Design review of the part built by this model. Coordinates are the model's own, in mm. A direction names the side the tool comes from. Round coordinates to 2 decimals unless told otherwise and drop trailing zeros. Loops run counter-clockwise (first coordinate to the right, second up) from the corner with the lowest first, then second, coordinate; pieces in that order, holes last. Notation, with made-up numbers: (56, 30) - (83, 30) arc R34 ccw to (83, 69) - close; hole circle Ø3 at (0, 39). An arc over 180 degrees is marked (long way). Use one line per item in the form item = value. Start each with the question number.
(1) We need section B-B, the plane z = 0. Write out the cut boundary in (x, y), then the cut area to 3 significant figures.
(2) We need section D-D, the plane y = 0.5. Write out the cut boundary in (x, z) (1 decimal), then the cut area to 3 significant figures.
(3) Wall thickness on probe 1 along Z at (x, y) = (6, -2.75) (3 decimals); probe 2 along Z at (x, y) = (1, -3) (3 decimals); probe 3 along X at (y, z) = (-4.25, 1): over which ranges is each line inside the solid? List them lowest first. Write a range as [from, to].
(4) For pin 1 (2 mm diameter, centred on y = -2.5, z = 6, fed in from +X); pin 2 (2 mm diameter, centred on x = 0, z = 0.5, fed in from -Y), all flat-tipped, find the tip position at first contact; note any pin that passes through.
(5) Machinability: for faces 1 (the cylindrical face through (12.362, -2.929, -7.521)), 2 (the flat face through (-12.588, -3, 0)), which of the approach directions +Z, -Z, +X, -X, +Y, -Y give a long, thin tool a straight path to every point of the face, cutting with its end or side? Answer none if there is none.
(6) The part is to be moulded in two halves that separate along X. For faces 3 (the flat face through (-1, -2, -0.6)), 4 (the flat face through (13.788, -3, 0)), 5 (the cylindrical face through (-13.186, 0.63, -0.056)), say which applies: released by +X, released by -X, zero draft, split by the parting line, or undercut.
(7) We need section A-A, the plane y = -3. Give the number of separate pieces and of enclosed holes in the cut face, then the cut area to 3 significant figures.
(8) We need section C-C, the plane x = 0. Write out the cut boundary in (y, z) (3 decimals).
from build123d import *

# Parameters (mm, degrees)
SKETCH_1_R      = 2.8
EXTRUDE_1_DEPTH = 5
SKETCH_2_W      = 27.575
SKETCH_2_H      = 18.05
EXTRUDE_2_DEPTH = 1.2
SKETCH_3_W      = 27.575
SKETCH_3_H      = 18.05
SKETCH_3_W_2    = 25.175
SKETCH_3_H_2    = 15.65
EXTRUDE_3_DEPTH = 5
FILLET_1_R      = 5
FILLET_2_R      = 2
CHAMFER_1_SIZE  = 0.5


with BuildPart() as part:
    # 草图1 → 凸台-拉伸1 (new body)
    with BuildSketch(Plane(origin=(0, 0, 0), x_dir=(1, 0, 0), z_dir=(0, 1, 0))):
        with Locations(Location((0, 0, 0), (0, 0, 270))):
            Circle(SKETCH_1_R)
        Polygon((2.2, 0.6), (2.2, -0.6), (0.6, -0.6), (0.6, -2.2), (-0.6, -2.2), (-0.6, -0.6), (-2.2, -0.6), (-2.2, 0.6), (-0.6, 0.6), (-0.6, 2.2), (0.6, 2.2), (0.6, 0.6), align=None, mode=Mode.SUBTRACT)
    extrude(amount=-EXTRUDE_1_DEPTH)

    # 草图2 → 凸台-拉伸2 (add)
    with BuildSketch(Plane(origin=(0, 0, 0), x_dir=(1, 0, 0), z_dir=(0, 1, 0))):
        Rectangle(SKETCH_2_W, SKETCH_2_H)
    extrude(amount=EXTRUDE_2_DEPTH)

    # 草图3 → 凸台-拉伸3 (add)
    with BuildSketch(Plane(origin=(0, 0, 0), x_dir=(1, 0, 0), z_dir=(0, 1, 0))):
        Rectangle(SKETCH_3_W, SKETCH_3_H)
        Rectangle(SKETCH_3_W_2, SKETCH_3_H_2, mode=Mode.SUBTRACT)
    extrude(amount=-EXTRUDE_3_DEPTH)

    # 圆角1
    fillet_1_edges = [part.edges().sort_by_distance(p)[0] for p in [
        (13.7875, -1.9, 9.025),
        (13.7875, -1.9, -9.025),
        (-13.7875, -1.9, -9.025),
        (-13.7875, -1.9, 9.025),
        (-12.5875, -2.5, 7.825),
        (-12.5875, -2.5, -7.825),
        (12.5875, -2.5, -7.825),
        (12.5875, -2.5, 7.825),
    ]]
    fillet(fillet_1_edges, radius=FILLET_1_R)

    # 圆角2
    fillet_2_edges = [part.edges().sort_by_distance(p)[0] for p in [
        (-12.5875, 0, 0),
        (0, 0, 7.825),
        (0, 0, -7.825),
        (12.5875, 0, 0),
        (-11.123033906, 0, 6.360533906),
        (11.123033906, 0, 6.360533906),
        (11.123033906, 0, -6.360533906),
        (-11.123033906, 0, -6.360533906),
        (0, 1.2, -9.025),
        (13.7875, 1.2, 0),
        (-13.7875, 1.2, 0),
        (0, 1.2, 9.025),
        (-12.323033906, 1.2, -7.560533906),
        (-12.323033906, 1.2, 7.560533906),
        (12.323033906, 1.2, 7.560533906),
        (12.323033906, 1.2, -7.560533906),
    ]]
    fillet(fillet_2_edges, radius=FILLET_2_R)

    # 倒角1
    chamfer_1_edges = [part.edges().sort_by_distance(p)[0] for p in [
        (0, 0, -2.8),
    ]]
    chamfer(chamfer_1_edges, length=CHAMFER_1_SIZE)


solid = part.part
Data:
q1.outline = (-13.79, -5) - (-12.59, -5) - (-12.59, -2) arc R2 cw to (-10.59, 0) - (-3.3, 0) - (-2.8, -0.5) - (-2.8, -5) - (-2.2, -5) - (-2.2, 0) - (2.2, 0) - (2.2, -5) - (2.8, -5) - (2.8, -0.5) - (3.3, 0) - (10.59, 0) arc R2 cw to (12.59, -2) - (12.59, -5) - (13.79, -5) - (13.79, -0.8) arc R2 ccw to (11.79, 1.2) - (-11.79, 1.2) arc R2 ccw to (-13.79, -0.8) - close
q1.area = 51.3 mm^2
q2.outline = (-13.3, -4) arc R4.5 ccw to (-8.8, -8.5) - (8.8, -8.5) arc R4.5 ccw to (13.3, -4) - (13.3, 4) arc R4.5 ccw to (8.8, 8.5) - (-8.8, 8.5) arc R4.5 ccw to (-13.3, 4) - close
q2.area = 437 mm^2
q3.probe_1 = [-9.025, -7.825], [7.825, 9.025]
q3.probe_2 = [-9.025, -7.825], [-2.615, -0.6], [0.6, 2.615], [7.825, 9.025]
q3.probe_3 = [-13.79, -12.59], [-2.62, -0.6], [0.6, 2.62], [12.59, 13.79]
q4.pin_1 = 13.69
q4.pin_2 = -5
q5.face_1 = -Z, +X, +Y, -Y
q5.face_2 = -Y
q6.face_3 = undercut
q6.face_4 = released by +X
q6.face_5 = released by -X
q7.separate_pieces = 2
q7.enclosed_holes = 2
q7.area = 119 mm^2
q8.outline = (-5, -9.025) - (-0.8, -9.025) arc R2 ccw to (1.2, -7.025) - (1.2, 7.025) arc R2 ccw to (-0.8, 9.025) - (-5, 9.025) - (-5, 7.825) - (-2, 7.825) arc R2 cw to (0, 5.825) - (0, 3.3) - (-0.5, 2.8) - (-5, 2.8) - (-5, 2.2) - (0, 2.2) - (0, -2.2) - (-5, -2.2) - (-5, -2.8) - (-0.5, -2.8) - (0, -3.3) - (0, -5.825) arc R2 cw to (-2, -7.825) - (-5, -7.825) - close
